```python
from build123d import *

# Parameters (mm, degrees)
EXTRUDE1_DEPTH                  = 19.05
F_4_40_TAPPED_HOLE1_D           = 2.2606
F_4_40_TAPPED_HOLE1_DEPTH       = 8.89
F_4_40_TAPPED_HOLE1_CBORE_D     = 2.8448
F_4_40_TAPPED_HOLE1_CBORE_DEPTH = 5.588
F_4_40_TAPPED_HOLE1_TIP         = 0.679152758


with BuildPart() as part:
    # Sketch1 → Extrude1 (new body, symmetric)
    with BuildSketch(Plane(origin=(0, 0, 0), x_dir=(1, 0, 0), z_dir=(0, 1, 0))):
        Polygon((-4.7625, -4.7625), (-1.5875, -4.7625), (-1.5875, 1.5875), (1.5875, 1.5875), (1.5875, -4.7625), (4.7625, -4.7625), (4.7625, 4.7625), (-4.7625, 4.7625), align=None)
    extrude(amount=EXTRUDE1_DEPTH, both=True)

    # #4-40 Tapped Hole1
    with Locations(Plane(origin=(0, 7.9375, -4.7625), x_dir=(-1, 0, 0), z_dir=(0, 0, -1))):
        with Locations((0, 0), (0, -22.225)):
            CounterBoreHole(F_4_40_TAPPED_HOLE1_D / 2, F_4_40_TAPPED_HOLE1_CBORE_D / 2, F_4_40_TAPPED_HOLE1_CBORE_DEPTH, depth=F_4_40_TAPPED_HOLE1_DEPTH)
            with Locations((0, 0, -(F_4_40_TAPPED_HOLE1_DEPTH + F_4_40_TAPPED_HOLE1_TIP / 2))):  # 118° drill point
                Cone(0, F_4_40_TAPPED_HOLE1_D / 2, F_4_40_TAPPED_HOLE1_TIP, mode=Mode.SUBTRACT)


solid = part.part
```
CAD build for the part. Positions are in the model's coordinates, mm. A direction names the side the tool comes from. Give positions to 0.01 mm unless a question says otherwise; leave off trailing zeros. Loops run counter-clockwise (first coordinate to the right, second up) from the corner with the lowest first, then second, coordinate; pieces in that order, holes last. Notation, with made-up numbers: M 6,79.25 L 33,79.25 A20 ccw 33,85.25 Z; hole C 3,9.25 d5. An arc over 180 degrees is marked long. Use one line per item in the form item = value.
Item 1: Slice it at A-A (x = 0). List the corners of the cut face in (y, z).
Determined:
outline = M -19.05,-4.76 L -15.71,-4.76 L -15.71,-1.59 L -19.05,-1.59 Z; M -12.87,-4.76 L 6.52,-4.76 L 6.52,-1.59 L -12.87,-1.59 Z; M 9.36,-4.76 L 19.05,-4.76 L 19.05,-1.59 L 9.36,-1.59 Z
Item 2: Flat gauge pin, fed straight in: pin 1 (2.5 mm diameter, centred on x = 0, y = -14.29, fed in from +Z). Where does the tip first touch, or does it go through?
Determined:
pin_1 = through
Item 3: Slice it at C-C (y = -4.5). List the corners of the cut face in (x, z).
Determined:
outline = M -4.76,-4.76 L 4.76,-4.76 L 4.76,4.76 L 1.59,4.76 L 1.59,-1.59 L -1.59,-1.59 L -1.59,4.76 L -4.76,4.76 Z
Item 4: Which spindle directions (+Z, -Z, +X, -X, +Y, -Y) get a long thin tool onto all of the face, cutting with end or side? Do faces 1 (the face through (4.762, 0, 0)), 2 (the face through (-1.588, 0, 2)). Say none if no direction does.
Determined:
face_1 = +Z, -Z, +X, +Y, -Y
face_2 = +Z, +Y, -Y
Item 5: Drill centre lines: probe 1 along Y at (x, z) = (0, -2.75); probe 2 along X at (y, z) = (15, 2.75); probe 3 along Z at (x, y) = (-1, 10). Where is each one in solid material? Low to high. Write a range as from..to.
Determined:
probe_1 = -19.05..-15.71, -12.87..6.52, 9.36..19.05
probe_2 = -4.76..-1.59, 1.59..4.76
probe_3 = -4.76..-1.59
Item 6: Slice it at B-B (z = -0.5). List the corners of the cut face in (x, y).
Determined:
outline = M -4.76,-19.05 L -1.59,-19.05 L -1.59,19.05 L -4.76,19.05 Z; M 1.59,-19.05 L 4.76,-19.05 L 4.76,19.05 L 1.59,19.05 Z
Item 7: Two-plate mould, pull along Y, no slides. Class faces 3 (the face through (0.31, 6.55, -3.2)), 4 (the face through (0, 19.05, -2)), 5 (the face through (0, 0, -4.762)): pulls with the +Y half, pulls with the -Y half, needs draft (parallel to the pull), parting line crosses it, or undercut.
Determined:
face_3 = undercut
face_4 = pulls with the +Y half
face_5 = needs draft
Item 8: Slice it at D-D (z = -3.5). List the corners of the cut face in (x, y), plus the area to 3 significant figures.
Determined:
outline = M -4.76,-19.05 L 4.76,-19.05 L 4.76,19.05 L -4.76,19.05 Z; hole C 0,-14.29 d2.84; hole C 0,7.94 d2.84
area = 350 mm2
